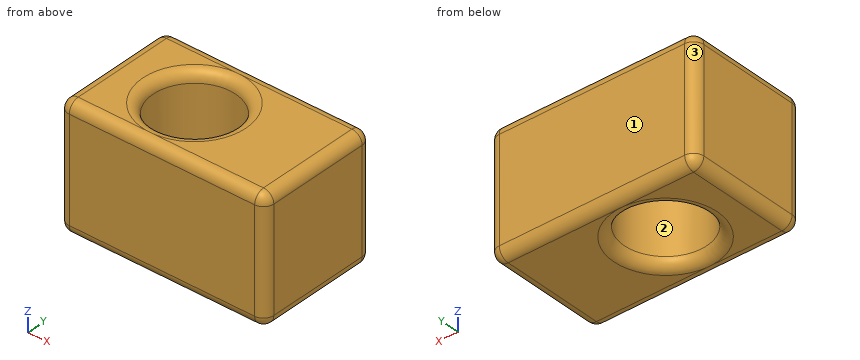
```python
from build123d import *

# Parameters (mm, degrees)
F0_W     = 101.6
F0_H     = 76.2
F0_R     = 25.4
F1_DEPTH = 38.1
F2_DEPTH = 25.4
F3_R     = 6.34999


# Not quite as in the source:
# - a fillet or chamfer is up to 0.001 mm smaller than in the source, because OpenCascade refuses the exact size


with BuildPart() as f1:
    # F0 (on Top) → F1 (new body, symmetric)
    with BuildSketch(Plane.XY):
        Rectangle(F0_W, F0_H)
        Circle(F0_R, mode=Mode.SUBTRACT)
    extrude(amount=F1_DEPTH, both=True)

    # F2 (add): a face of the model
    f2_faces = [f1.faces().sort_by_distance(p)[0] for p in [
        (50.8, 0, 0),
    ]]
    extrude(f2_faces, amount=F2_DEPTH)

    # F3 (radius 6.35 in the source; OpenCascade refuses exactly that, so slightly less here)
    f3_edges = [f1.edges().sort_by_distance(p)[0] for p in [
        (12.7, 38.1, 38.1),
        (-50.8, 0, 38.1),
        (12.7, -38.1, 38.1),
        (76.2, 0, 38.1),
        (-25.4, 0, 38.1),
        (-50.8, 38.1, 0),
        (-50.8, 0, -38.1),
        (-50.8, -38.1, 0),
        (76.2, 38.1, 0),
        (12.7, 38.1, -38.1),
        (12.7, -38.1, -38.1),
        (76.2, -38.1, 0),
        (76.2, 0, -38.1),
        (-25.4, 0, -38.1),
    ]]
    fillet(f3_edges, radius=F3_R)


solid = f1.part
```
CAD build for the part. Positions are in the model's coordinates, mm. Face numbers are marked on the shaded views. Coordinates: 2 decimals unless noted, no trailing zeros. Order: outer loops, then holes, each group sorted by start corner. A loop starts at its lowest first (then second) coordinate and runs counter-clockwise, first axis right, second up.
(1) Drill centre lines: L1, parallel to Y at x = 0, z = -14; L2, parallel to Z at x = 9, y = -30; L3, parallel to X at y = -6, z = -30.5. Where is each one in solid material? Low to high.
Solution:
L1: y = -38.1 to -25.4, 25.4 to 38.1
L2: z = -38.09 to 38.09
L3: x = -50.8 to -24.68, 24.68 to 76.2
(2) Saw through at C-C, the plane z = 26.5. Write the cut outline in (x, y).
Solution:
outline: (-50.8, -31.75) arc R6.35 ccw to (-44.45, -38.1) - (69.85, -38.1) arc R6.35 ccw to (76.2, -31.75) - (76.2, 31.75) arc R6.35 ccw to (69.85, 38.1) - (-44.45, 38.1) arc R6.35 ccw to (-50.8, 31.75) - close; hole circle Ø50.8 at (0, 0)
(3) Mould opens along X. For the marked faces 1, 2 and 3 say: released by +X, released by -X, zero draft, split by the parting line, or undercut.
Solution:
face 1: zero draft
face 2: undercut
face 3: released by -X
(4) Saw through at B-B, the plane y = 0. Write the cut outline in (x, z).
Solution:
outline: (-50.8, -31.75) arc R6.35 ccw to (-44.45, -38.1) - (-31.75, -38.1) arc R6.35 ccw to (-25.4, -31.75) - (-25.4, 31.75) arc R6.35 ccw to (-31.75, 38.1) - (-44.45, 38.1) arc R6.35 ccw to (-50.8, 31.75) - close; (25.4, -31.75) arc R6.35 ccw to (31.75, -38.1) - (69.85, -38.1) arc R6.35 ccw to (76.2, -31.75) - (76.2, 31.75) arc R6.35 ccw to (69.85, 38.1) - (31.75, 38.1) arc R6.35 ccw to (25.4, 31.75) - close
